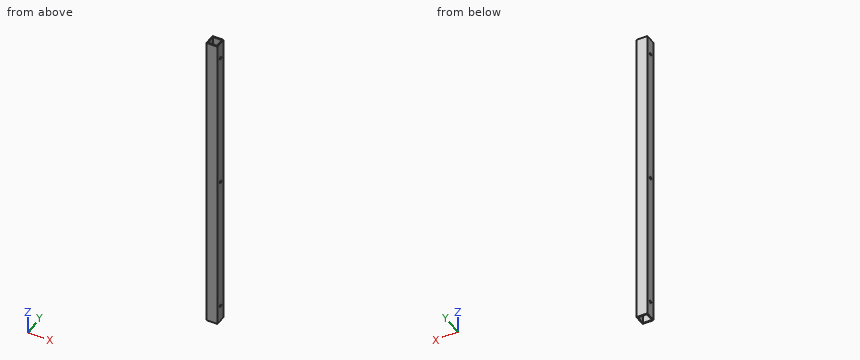
from build123d import *

# Parameters (mm, degrees)
SKETCH_1_W          = 20
SKETCH_1_H          = 20
SKETCH_1_W_2        = 16
SKETCH_1_H_2        = 16
EXTRUDE_1_DEPTH     = 560
SKETCH_2_R          = 2.5
CUT_EXTRUDE_1_DEPTH = 20


with BuildPart() as part:
    # 草图1 → 凸台-拉伸1 (new body)
    with BuildSketch(Plane.XY):
        Rectangle(SKETCH_1_W, SKETCH_1_H)
        Rectangle(SKETCH_1_W_2, SKETCH_1_H_2, mode=Mode.SUBTRACT)
    extrude(amount=-EXTRUDE_1_DEPTH)

    # 草图2 → 切除-拉伸1 (cut)
    with BuildSketch(Plane(origin=(10, 0, 0), x_dir=(0, 0, -1), z_dir=(1, 0, 0))):
        with Locations((280, 0)):
            Circle(SKETCH_2_R)
        with Locations((30, 0)):
            Circle(SKETCH_2_R)
        with Locations((530, 0)):
            Circle(SKETCH_2_R)
    extrude(amount=-CUT_EXTRUDE_1_DEPTH, mode=Mode.SUBTRACT)


solid = part.part
Could you check a few things on this model? Use its own coordinates, in mm. Coordinates: 2 decimals unless noted, no trailing zeros. Order: outer loops, then holes, each group sorted by start corner. A loop starts at its lowest first (then second) coordinate and runs counter-clockwise, first axis right, second up.
Q1. Please list where these lines run through material, in increasing order: L1, parallel to Y at x = -2.5, z = -139; L2, parallel to Y at x = -8.9, z = -30.
Q2. Suppose I cut it at A-A on x = -4. Please give me the cut outline in (y, z).
Q3. Will this pin go through, and if not, where does the flat tip stop? pin 1 (4 mm diameter, centred on y = 0, z = -30, fed in from -X).
Answer:
1. L1: y = -10 to -8, 8 to 10
1. L2: y = -10 to -2.5, 2.5 to 10
2. outline: (-10, -560) - (-8, -560) - (-8, 0) - (-10, 0) - close; (8, -560) - (10, -560) - (10, 0) - (8, 0) - close
3. pin 1: passes through
